```python
from build123d import *

# Parameters (mm, degrees)
F1_DEPTH      = 10.16
F1_DEPTH_BACK = 10.16
F2_W          = 20.32
F2_H          = 35.56
F2_R          = 2.5781
F3_DEPTH      = 25.4
F4_W          = 14.224
F4_H          = 35.56
F5_DEPTH      = 54.61
F7_DEPTH      = 25.4


with BuildPart() as f1:
    # F0 (on Right) → F1 (new body, two sides)
    with BuildSketch(Plane.YZ) as f1_sk:
        with BuildLine():
            Line((-12.7, 0), (0, 0))
            Line((0, 0), (0, 66.04))
            ThreePointArc((0, 66.04), (-26.67, 70.940694), (-53.34, 66.04))
            Line((-53.34, 66.04), (-53.34, 27.94))
            ThreePointArc((-53.34, 27.94), (-48.702079, 19.030695), (-38.743793, 17.719745))
            ThreePointArc((-38.743793, 17.719745), (-38.570599, 17.787128), (-38.396755, 17.852819))
            ThreePointArc((-38.396755, 17.852819), (-20.880736, 15.644858), (-12.7, 0))
        make_face()
    extrude(amount=F1_DEPTH)
    extrude(f1_sk.sketch, amount=-F1_DEPTH_BACK)

    # F2 (on face) → F3 (cut)
    with BuildSketch(Plane.YZ.offset(10.16)):
        with Locations((-21.336, 48.26)):
            Rectangle(F2_W, F2_H)
        with Locations((-44.704, 27.94)):
            Circle(F2_R)
    extrude(amount=-F3_DEPTH, mode=Mode.SUBTRACT)

    # F4 (on face) → F5 (cut)
    with BuildSketch(Plane(origin=(0, 0, 0), x_dir=(-1, 0, 0), z_dir=(0, 1, 0))):
        with BuildLine():
            Line((7.112, 43.021353), (7.112, 62.134647))
            ThreePointArc((7.112, 62.134647), (0, 64.4906), (-7.112, 62.134647))
            Line((-7.112, 62.134647), (-7.112, 43.021353))
            ThreePointArc((-7.112, 43.021353), (0, 40.6654), (7.112, 43.021353))
        make_face()
        with Locations((0, 20.828)):
            Rectangle(F4_W, F4_H)
    extrude(amount=-F5_DEPTH, mode=Mode.SUBTRACT)

    # F6 (on face) → F7 (cut)
    with BuildSketch(Plane.XZ.offset(53.34)):
        with BuildLine():
            Line((-7.112, 43.443549), (-7.112, 38.608))
            Line((-7.112, 38.608), (7.112, 38.608))
            Line((7.112, 38.608), (7.112, 43.443549))
            ThreePointArc((7.112, 43.443549), (0, 41.004444), (-7.112, 43.443549))
        make_face()
    extrude(amount=-F7_DEPTH, mode=Mode.SUBTRACT)


solid = f1.part
```
Geometry: final body of the model. Coordinates: model frame, mm. A direction names the side the tool comes from. Round coordinates to 2 decimals unless told otherwise and drop trailing zeros. Order: outer loops, then holes, each group sorted by start corner. A loop starts at its lowest first (then second) coordinate and runs counter-clockwise, first axis right, second up. Notation, with made-up numbers: (14.25, 80) -> (67.25, 80) arc R26 ccw to (67.25, 119) -> close; hole circle Ø5 at (17, -6). An arc over 180 degrees is marked (long way). Use CSV: the item, a comma, the result in double quotes. Start each with the question number.
1) Section B-B (x = -3). Return the cut outline in (y, z).
2) Section D-D (z = 20.5). Return the cut outline in (x, y).
3) Set-up query: faces 4 (the face through (-7.5, -31.496, 48.2)), 5 (the face through (0.107, -5.51, 40.666)), 6 (the face through (-0.11, -42.27, 64.49)). Return all of +Z, -Z, +X, -X, +Y, -Y with unobstructed straight access to the full face (end or side cutting, diameter ignored); none if empty.
4) Section A-A (z = 61). Return the cut outline in (x, y), and give its area (3 significant figures).
5) First-contact query: pin 1 Ø10 at (x, y) = (0, -25) entering from -Z; pin 2 Ø10.5 at (x, y) = (-2.5, -6) entering from +Z; pin 3 Ø6 at (x, y) = (-6, -18.5) entering from +Z. Flat tips, straight axial feed; report the tip coordinate or a pass-through.
6) Draft query along Y for faces 1 (the face through (-7.5, 0, 32.9)), 2 (the face through (0, -6, 3.048)), 3 (the face through (0, -21, 66.04)). Return one class per face: +Y half, -Y half, draft (parallel to the pull), parting line (faces both ways), or undercut.
7) Section C-C (y = -46). Return the cut outline in (x, z).
8) Material intervals for line 1 along X through (y, z) = (-2.5, 30); line 2 along Y through (x, z) = (8.5, 65.5); line 3 along Z through (x, y) = (7.5, -21), sorted ascending. Write a range as from..to.
Returned:
1,outline,"(-53.34, 64.11) -> (-31.5, 64.11) -> (-31.5, 66.04) -> (-11.18, 66.04) -> (-11.18, 64.11) -> (0, 64.11) -> (0, 66.04) arc R75.02 ccw to (-53.34, 66.04) -> close; (-12.95, 3.05) arc R19.05 cw to (-12.7, 0) -> (0, 0) -> (0, 3.05) -> close; (-11.18, 38.61) -> (0, 38.61) -> (0, 41.05) -> (-11.18, 41.05) -> close"
2,outline,"(-10.16, -50.4) -> (-7.11, -50.4) -> (-7.11, 0) -> (-10.16, 0) -> close; (7.11, -50.4) -> (10.16, -50.4) -> (10.16, 0) -> (7.11, 0) -> close"
3,face 4,"+X, -X"
3,face 5,"+Y, -Y"
3,face 6,"-Z, +Y, -Y"
4,outline,"(-10.16, -53.34) -> (-7.11, -53.34) -> (-7.11, -31.5) -> (-10.16, -31.5) -> close; (-10.16, -11.18) -> (-7.11, -11.18) -> (-7.11, 0) -> (-10.16, 0) -> close; (7.11, -53.34) -> (10.16, -53.34) -> (10.16, -31.5) -> (7.11, -31.5) -> close; (7.11, -11.18) -> (10.16, -11.18) -> (10.16, 0) -> (7.11, 0) -> close"
4,area,"201 mm²"
5,pin 1,"stops at z = 66.04"
5,pin 2,"stops at z = 69.34"
5,pin 3,"stops at z = 70.76"
6,face 1,"+Y half"
6,face 2,"draft"
6,face 3,"undercut"
7,outline,"(-10.16, 17.65) -> (-7.11, 17.65) -> (-7.11, 25.71) -> (-10.16, 25.71) -> close; (-10.16, 30.17) -> (-7.11, 30.17) -> (-7.11, 62.13) arc R11.91 cw to (7.11, 62.13) -> (7.11, 30.17) -> (10.16, 30.17) -> (10.16, 68.41) -> (-10.16, 68.41) -> close; (7.11, 17.65) -> (10.16, 17.65) -> (10.16, 25.71) -> (7.11, 25.71) -> close"
8,line 1,"x = -10.16..-7.11, 7.11..10.16"
8,line 2,"y = -53.34..-31.5, -11.18..0"
8,line 3,"z = 15.73..30.48, 66.04..70.73"
